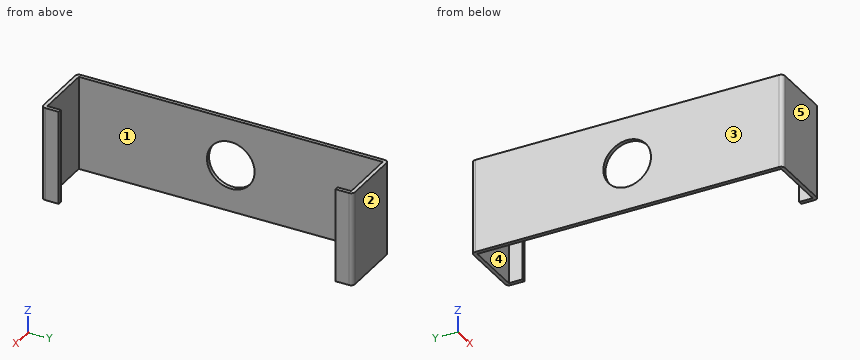
from build123d import *

# Parameters (mm, degrees)
SKETCH1_W                 = 15.494
SKETCH1_H                 = 3.175
BASE_FLANGE1_DEPTH        = 0.127
SKETCHED_START            = -1.5875
SKETCHED_BEND16_DEPTH     = 3.175
SKETCHED_BEND16_2_DEPTH   = 3.175
F_0_CLEARANCE_HOLE1_D     = 1.6129
F_0_CLEARANCE_HOLE1_DEPTH = 4.826
F_0_CLEARANCE_HOLE1_TIP   = 0.484564046


# Read off the part's stored shape, not the designer's step: Sketched Bend16
# Sheet-metal steps are written as plain solids
with BuildPart() as part:
    # Sketch1 → Base-Flange1 (new body)
    with BuildSketch(Plane(origin=(0, 0, 0), x_dir=(1, 0, 0), z_dir=(0, 1, 0))):
        Rectangle(SKETCH1_W, SKETCH1_H)
    extrude(amount=-BASE_FLANGE1_DEPTH)

    # Sketched Bend16 outline → Sketched Bend16 (cut)
    with BuildSketch(Plane.XY.offset(SKETCHED_START)):
        with BuildLine():
            ThreePointArc((5.246167695, -0.127), (5.155471554, -0.089952279), (5.116652599, 0))
            Line((5.116652599, 0), (-7.747, 0))
            Line((-7.747, 0), (-7.747, -0.127))
            Line((-7.747, -0.127), (5.246167695, -0.127))
        make_face()
        with BuildLine():
            Line((7.747, 0), (7.316647401, 0))
            ThreePointArc((7.316647401, 0), (7.277828446, -0.089952279), (7.187132305, -0.127))
            Line((7.187132305, -0.127), (7.747, -0.127))
            Line((7.747, -0.127), (7.747, 0))
        make_face()
    extrude(amount=SKETCHED_BEND16_DEPTH, mode=Mode.SUBTRACT)

    # Sketched Bend16 2 outline → Sketched Bend16 2 (add)
    with BuildSketch(Plane.XY.offset(SKETCHED_START)):
        with BuildLine():
            Line((5.243627695, 0.00254), (5.243627695, 10.287404611))
            ThreePointArc((5.243627695, 10.287404611), (5.244371643, 10.289200662), (5.246167695, 10.289944611))
            Line((5.246167695, 10.289944611), (7.187132305, 10.289944611))
            ThreePointArc((7.187132305, 10.289944611), (7.188928357, 10.289200662), (7.189672305, 10.287404611))
            Line((7.189672305, 10.287404611), (7.189672305, 9.831272305))
            Line((7.189672305, 9.831272305), (7.316672305, 9.831272305))
            Line((7.316672305, 9.831272305), (7.316672305, 10.287404611))
            ThreePointArc((7.316672305, 10.287404611), (7.278730917, 10.379003223), (7.187132305, 10.416944611))
            Line((7.187132305, 10.416944611), (5.246167695, 10.416944611))
            ThreePointArc((5.246167695, 10.416944611), (5.154569083, 10.379003223), (5.116627695, 10.287404611))
            Line((5.116627695, 10.287404611), (5.116627695, 0.00254))
            ThreePointArc((5.116627695, 0.00254), (5.116633921, 0.001269939), (5.116652599, 0))
            Line((5.116652599, 0), (5.246167695, 0))
            ThreePointArc((5.246167695, 0), (5.244371644, 0.000743949), (5.243627695, 0.00254))
        make_face()
        with BuildLine():
            ThreePointArc((7.189672305, 0.00254), (7.188928356, 0.000743949), (7.187132305, 0))
            Line((7.187132305, 0), (7.316647401, 0))
            ThreePointArc((7.316647401, 0), (7.316666079, 0.001269939), (7.316672305, 0.00254))
            Line((7.316672305, 0.00254), (7.316672305, 0.458672305))
            Line((7.316672305, 0.458672305), (7.189672305, 0.458672305))
            Line((7.189672305, 0.458672305), (7.189672305, 0.00254))
        make_face()
    extrude(amount=SKETCHED_BEND16_2_DEPTH)

    # #0 Clearance Hole1
    with Locations(Plane(origin=(5.243627695, 0, 0), x_dir=(0, 0, -1), z_dir=(1, 0, 0))):
        with Locations((0, 5.144972305)):
            Hole(F_0_CLEARANCE_HOLE1_D / 2, depth=F_0_CLEARANCE_HOLE1_DEPTH)
            with Locations((0, 0, -(F_0_CLEARANCE_HOLE1_DEPTH + F_0_CLEARANCE_HOLE1_TIP / 2))):  # 118° drill point
                Cone(0, F_0_CLEARANCE_HOLE1_D / 2, F_0_CLEARANCE_HOLE1_TIP, mode=Mode.SUBTRACT)


solid = part.part
The listing builds one solid part. Answer for the finished solid, in the listing's coordinates (mm). Face numbers are marked on the shaded views. A direction names the side the tool comes from. Give positions to 0.01 mm unless a question says otherwise; leave off trailing zeros. Order: outer loops, then holes, each group sorted by start corner. A loop starts at its lowest first (then second) coordinate and runs counter-clockwise, first axis right, second up. Notation, with made-up numbers: (13.25, 51.5) -> (57.25, 51.5) arc R23 ccw to (57.25, 83.5) -> close; hole circle Ø3 at (-33, 11.25). An arc over 180 degrees is marked (long way). Put each result on its own line as item: value.
Item 1: Given P1, Ø1.9, axis at y = 5.14, z = 0, coming from the +X side, flat-ended and moving along its own axis, determine where the tip first touches the part or whether it passes through.
Established:
P1: stops at x = 5.24
Item 2: A cutting plane is placed at C-C on y = 5.5. Give the vertices of the cut face in (x, z).
Established:
outline: (5.12, -1.59) -> (5.24, -1.59) -> (5.24, -0.72) -> (5.12, -0.72) -> close; (5.12, 0.72) -> (5.24, 0.72) -> (5.24, 1.59) -> (5.12, 1.59) -> close
Item 3: A straight line is drawn through the part: line 1 (Y direction, x = 5.2, z = 0). Find the intervals that lie inside material, in ascending order.
Established:
line 1: y = -0.12 to 4.34, 5.95 to 10.41
Item 4: For a pull along Y with two mould halves and no side action, classify the marked faces 1, 2 and 3 as released by +Y, released by -Y, zero draft, split by the parting line, or undercut.
Established:
face 1: undercut
face 2: released by +Y
face 3: zero draft
Item 5: A cutting plane is placed at A-A on x = 6.95. Give the vertices of the cut face in (y, z), plus the area to 3 significant figures.
Established:
outline: (-0.13, -1.59) -> (0, -1.59) -> (0, 1.59) -> (-0.13, 1.59) -> close; (10.29, -1.59) -> (10.42, -1.59) -> (10.42, 1.59) -> (10.29, 1.59) -> close
area: 0.806 mm^2
Item 6: For the marked faces 4 and 5, determine the directions among +Z, -Z, +X, -X, +Y, -Y from which every point of the face is accessible in a straight line to the end or side of a thin tool.
Established:
face 4: +Z, -Z
face 5: +Z, -Z, +X, -X, -Y
